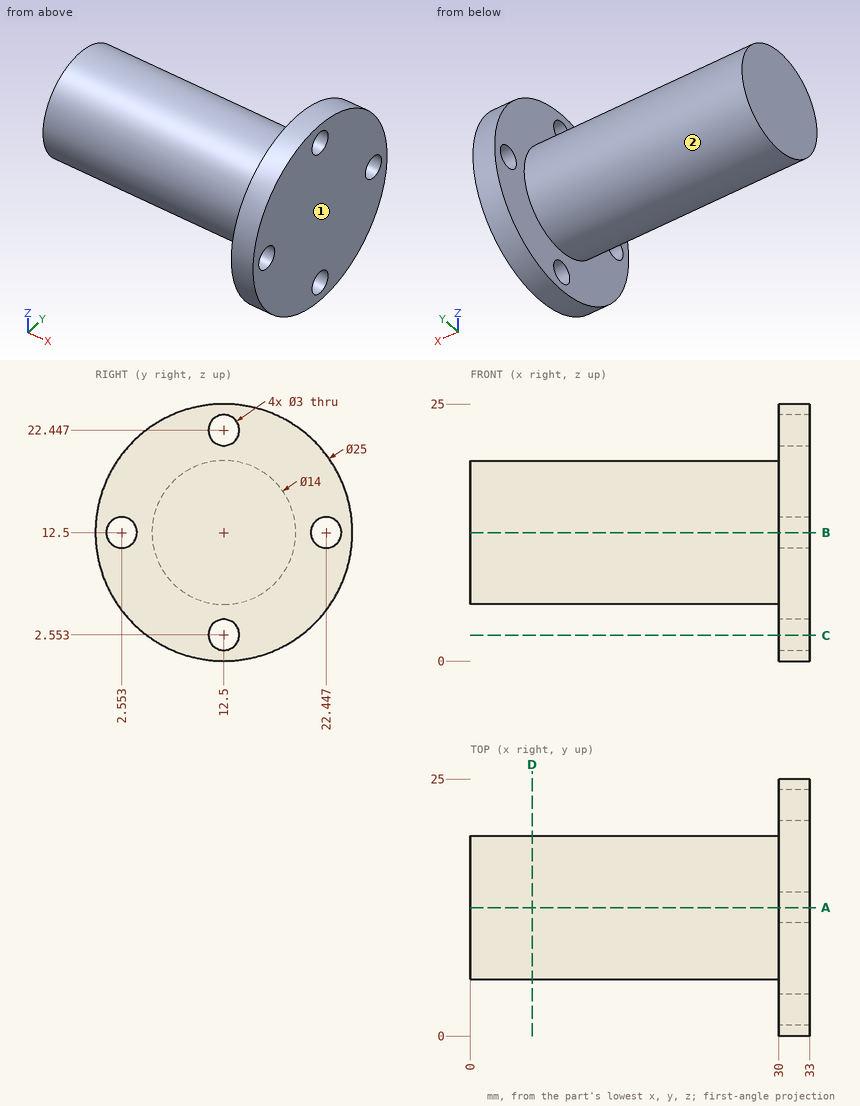
Geometry: see drawing. Coordinates: mm, zero at the bounding-box minimum. A direction names the side the tool comes from. Give positions to 0.01 mm unless a question says otherwise; leave off trailing zeros. Loops run counter-clockwise (first coordinate to the right, second up) from the corner with the lowest first, then second, coordinate; pieces in that order, holes last. Notation, with made-up numbers: (-3.75, -32.5) -> (54.25, -32.5) arc R38 ccw to (54.25, 6.5) -> close; hole circle Ø5 at (0, 32.5). An arc over 180 degrees is marked (long way). Use one line per item in the form item = value.
Item 1: Pin query (flat end, axial travel): P1, Ø8, axis at x = 10.5, z = 10, coming from the +Y side; P2, Ø2.5, axis at y = 12.5, z = 22.45, coming from the -X side; P3, Ø12, axis at x = 10, z = 9, coming from the -Y side; P4, Ø4, axis at x = 11, y = 12, coming from the +Z side. Return the tip coordinate at first contact, or that it passes through.
A:
P1 = 19.5
P2 = through
P3 = 5.5
P4 = 19.5
Item 2: Section query D-D on x = 6. Output: boundary loops of the cut face in (y, z), and give its area (3 significant figures).
A:
outline = circle Ø14 at (12.5, 12.5)
area = 154 mm^2
Item 3: Section query C-C on z = 2.5. Output: boundary loops of the cut face in (x, y).
A:
outline = (30, 5) -> (33, 5) -> (33, 11) -> (30, 11) -> close; (30, 14) -> (33, 14) -> (33, 20) -> (30, 20) -> close
Item 4: Access query for the marked faces 1 and 2. Directions: +Z, -Z, +X, -X, +Y, -Y. A direction counts if a zero-diameter tool reaches every point of the face in a straight line with its end or side. Return the directions, or none.
A:
face_1 = +Z, -Z, +X, +Y, -Y
face_2 = -X
Item 5: Section query A-A on y = 12.5. Output: boundary loops of the cut face in (x, z).
A:
outline = (0, 5.5) -> (30, 5.5) -> (30, 4.05) -> (33, 4.05) -> (33, 20.95) -> (30, 20.95) -> (30, 19.5) -> (0, 19.5) -> close; (30, 0) -> (33, 0) -> (33, 1.05) -> (30, 1.05) -> close; (30, 23.95) -> (33, 23.95) -> (33, 25) -> (30, 25) -> close
Item 6: Line query: probe 1 along Y at (x, z) = (31.6, 12.5); probe 2 along X at (y, z) = (4.75, 5.5); probe 3 along Y at (x, z) = (2, 12). Output: solid intervals per line, ascending.
A:
probe_1 = 0 to 1.05, 4.05 to 20.95, 23.95 to 25
probe_2 = 30 to 33
probe_3 = 5.52 to 19.48
